from build123d import *

# Parameters (mm, degrees)
POCKET_DEPTH = 20
CHAMFER_SIZE = 7


with BuildPart() as part:
    # Sketch → Revolution (revolve)
    with BuildSketch(Plane.XZ):
        Polygon((0, 0), (0, 15), (3.75, 15), (3.75, 3), (56.757359, 3), (58.757359, 1), (61.242641, 1), (63.242641, 3), (96.585786, 3), (98, 4.414214), (98, 20), (100, 20), (100, 0), align=None)
    revolve(axis=Axis((0, 0, 0), (0, 0, 1)))

    # Sketch001 (on DatumPlane) → Pocket (cut)
    with BuildSketch(Plane(origin=(0, 0, 4), x_dir=(-1, 0, 0), z_dir=(0, 0, 1))):
        with BuildLine():
            ThreePointArc((-60, -103.923048), (0, -120), (60, -103.923048))
            Line((32.5, -56.291651), (60, -103.923048))
            ThreePointArc((-32.5, -56.291651), (0, -65), (32.5, -56.291651))
            Line((-32.5, -56.291651), (-60, -103.923048))
        make_face()
    extrude(amount=POCKET_DEPTH, mode=Mode.SUBTRACT)

    # Chamfer
    chamfer_edges = [part.edges().sort_by_distance(p)[0] for p in [
        (-49.396447, 85.557155, 4),
        (49.396447, 85.557155, 4),
    ]]
    chamfer(chamfer_edges, length=CHAMFER_SIZE)


solid = part.part
Could you check a few things on this model? Use its own coordinates, in mm. A direction names the side the tool comes from. Round coordinates to 2 decimals unless told otherwise and drop trailing zeros. Write each loop counter-clockwise with the first axis right and the second up, starting at its lowest first coordinate (ties: lowest second). Pieces come first, ordered by that corner, then holes. Notation, with made-up numbers: (51, 73) - (90, 73) arc R28 cw to (90, 100) - close; hole circle Ø4 at (34, -6). An arc over 180 degrees is marked (long way). Put each result on its own line as item: value. Start each with the question number.
(1) I need wall thicknesses on probe 1 along Y at (x, z) = (0, 8.5); probe 2 along Z at (x, y) = (0, 6); probe 3 along X at (y, z) = (-72, 16.5). Which ranges of each line are inside material? Lowest first, please.
(2) I want a section at B-B, the plane y = 0. Please give me the cut outline in (x, z), plus the area to 3 significant figures.
(3) For faces 5 (the flat face through (46.48, 87.41, 7.55)), 6 (the cylindrical face through (-3.68, -97.93, 12.32)), 7 (the flat face through (-1, 1, 0)), which set-ups out of +Z, -Z, +X, -X, +Y, -Y let a thin tool reach every point of the face, with its end or its side?
(4) Will these pins go through, and if not, where does the flat tip stop? pin 1 (1.5 mm diameter, centred on x = -78, z = 6.5, fed in from -Y); pin 2 (3.5 mm diameter, centred on x = -2.5, y = 93.5, fed in from +Z); pin 3 (8 mm diameter, centred on y = 53, z = 14.5, fed in from +X).
(5) Thinking about a two-plate mould opening in Y: for faces 1 (the flat face through (0, 0, 15)), 2 (the flat face through (-46.399, 87.463, 7.451)), 3 (the flat face through (-12, 1, 3)), 4 (the cylindrical face through (-21.68, -97.62, 9.86)), which applies, released by +Y, released by -Y, zero draft, split by the parting line, or undercut?
(6) I want a section at A-A, the plane x = 0. Please give me the cut outline in (y, z), plus the area to 3 significant figures.
Here are the results:
1. probe 1: y = -100 to -98, -3.75 to 3.75
1. probe 2: z = 0 to 3
1. probe 3: x = -69.4 to -66.48, 66.48 to 69.4
2. outline: (-100, 0) - (100, 0) - (100, 20) - (98, 20) - (98, 4.41) - (96.59, 3) - (63.24, 3) - (61.24, 1) - (58.76, 1) - (56.76, 3) - (3.75, 3) - (3.75, 15) - (-3.75, 15) - (-3.75, 3) - (-56.76, 3) - (-58.76, 1) - (-61.24, 1) - (-63.24, 3) - (-96.59, 3) - (-98, 4.41) - (-98, 20) - (-100, 20) - close
2. area: 742 mm^2
3. face 5: +Z, +Y
3. face 6: +Z
3. face 7: -Z, +X, -X, +Y, -Y
4. pin 1: stops at y = -63.5
4. pin 2: stops at z = 3
4. pin 3: stops at x = 87.17
5. face 1: zero draft
5. face 2: released by +Y
5. face 3: undercut
5. face 4: split by the parting line
6. outline: (-100, 0) - (100, 0) - (100, 4) - (97.59, 4) - (96.59, 3) - (63.24, 3) - (61.24, 1) - (58.76, 1) - (56.76, 3) - (3.75, 3) - (3.75, 15) - (-3.75, 15) - (-3.75, 3) - (-56.76, 3) - (-58.76, 1) - (-61.24, 1) - (-63.24, 3) - (-96.59, 3) - (-98, 4.41) - (-98, 20) - (-100, 20) - close
6. area: 710 mm^2
